```python
from build123d import *

# Parameters (mm, degrees)
F1_DEPTH = 63.5
F2_DEPTH = 25.4
F3_DEPTH = 7.9375
F5_R     = 6.35
F6_R     = 6.35
F7_R     = 6.35
F8_R     = 6.35


with BuildPart() as f1:
    # F0 (on Front) → F1 (new body, symmetric)
    with BuildSketch(Plane.XZ):
        Polygon((22.225, 9.525), (-41.275, 9.525), (-41.275, -9.525), (41.275, -9.525), (41.275, 9.525), align=None)
    extrude(amount=F1_DEPTH, both=True)

    # F0 (on Front) → F2 (join, symmetric)
    with BuildSketch(Plane.XZ):
        with BuildLine():
            Line((22.225, 27.32094), (22.225, 9.525))
            Line((22.225, 9.525), (41.275, 9.525))
            Line((41.275, 9.525), (41.275, 27.32094))
            ThreePointArc((41.275, 27.32094), (47.109768, 39.617662), (60.325, 42.8752))
            Line((60.325, 42.8752), (60.325, 61.857935))
            add(Edge.make_bspline(
                [(48.832623, 61.241094), (52.4914, 61.474881), (56.318798, 61.67946), (60.325, 61.857935)],
                knots=[108.446727, 108.446727, 108.446727, 108.446727, 114.871759, 114.871759, 114.871759, 114.871759], degree=3))
            ThreePointArc((48.832623, 61.241094), (29.670553, 48.876348), (22.225, 27.32094))
        make_face()
        with BuildLine():
            add(Edge.make_bspline(
                [(60.325, 61.857935), (60.837854, 61.880782), (61.353639, 61.903202), (61.872375, 61.9252)],
                knots=[114.871759, 114.871759, 114.871759, 114.871759, 115.69426, 115.69426, 115.69426, 115.69426], degree=3))
            Line((60.325, 61.857935), (60.325, 42.8752))
            Line((60.325, 42.8752), (85.725, 42.8752))
            Line((85.725, 42.8752), (85.725, 61.9252))
            Line((85.725, 61.9252), (61.872375, 61.9252))
        make_face()
    extrude(amount=F2_DEPTH, both=True)

    # F0 (on Front) → F3 (join, symmetric)
    with BuildSketch(Plane.XZ):
        with BuildLine():
            add(Edge.make_bspline(
                [(-41.275, 9.525), (-26.639564, 45.028193), (-12.923076, 57.295065), (48.832623, 61.241094)],
                knots=[0, 0, 0, 0, 108.446727, 108.446727, 108.446727, 108.446727], degree=3))
            Line((-41.275, 9.525), (22.225, 9.525))
            Line((22.225, 9.525), (22.225, 27.32094))
            ThreePointArc((22.225, 27.32094), (29.670553, 48.876348), (48.832623, 61.241094))
        make_face()
    extrude(amount=F3_DEPTH, both=True)

    # F0 (on Front) → F4 (revolve)
    with BuildSketch(Plane.XZ):
        Polygon((111.125, 66.675), (85.725, 66.675), (85.725, 61.9252), (85.725, 42.8752), (85.725, 38.1), (111.125, 38.1), align=None)
    revolve(axis=Axis((85.725, 0, 52.3875), (0, 0, 1)))

    # F5
    f5_edges = [f1.edges().sort_by_distance(p)[0] for p in [
        (41.275, -63.5, 0),
    ]]
    fillet(f5_edges, radius=F5_R)

    # F6
    f6_edges = [f1.edges().sort_by_distance(p)[0] for p in [
        (-41.275, -63.5, 0),
    ]]
    fillet(f6_edges, radius=F6_R)

    # F7
    f7_edges = [f1.edges().sort_by_distance(p)[0] for p in [
        (-41.275, 63.5, 0),
    ]]
    fillet(f7_edges, radius=F7_R)

    # F8
    f8_edges = [f1.edges().sort_by_distance(p)[0] for p in [
        (41.275, 63.5, 0),
    ]]
    fillet(f8_edges, radius=F8_R)


solid = f1.part
```
The listing builds one solid part. Answer for the finished solid, in the listing's coordinates (mm). A direction names the side the tool comes from. Give positions to 0.01 mm unless a question says otherwise; leave off trailing zeros. Loops run counter-clockwise (first coordinate to the right, second up) from the corner with the lowest first, then second, coordinate; pieces in that order, holes last. Notation, with made-up numbers: M 3,77 L 53,77 A21 ccw 53,85 Z; hole C 36.5,64 d8. An arc over 180 degrees is marked long. One line per item, written item: value.
Q1. Find the intervals of material crossed by line 1 (Z direction, x = 72, y = -22); line 2 (Y direction, x = -11, z = 31.5); line 3 (Y direction, x = 61, z = 53), in increasing order. Write a range as from..to.
Working result:
line 1: z = 42.88..61.93
line 2: y = -7.94..7.94
line 3: y = -25.4..25.4
Q2. For faces 1 (the face through (46, 25.4, 42)), 2 (the face through (29.87, 16.55, 49.13)), 3 (the face through (29.87, -16.79, 49.13)), 4 (the face through (46, -25.4, 42)), 5 (the face through (41.275, -1, 5)), determine the directions among +Z, -Z, +X, -X, +Y, -Y from which every point of the face is accessible in a straight line to the end or side of a thin tool.
Working result:
face 1: +Z, +X, -X, +Y
face 2: +Z, -X, +Y
face 3: +Z, -X, -Y
face 4: +Z, +X, -X, -Y
face 5: -Z, +X, +Y, -Y
Q3. Flat-ended cylindrical pins translate along their axes: P1, Ø15, axis at x = 94.5, y = -1.5, coming from the -Z side; P2, Ø6, axis at x = 24.5, y = -44, coming from the +Z side (3 decimals); P3, Ø15.5, axis at x = 69, z = 40.5, coming from the +Y side; P4, Ø19, axis at y = -16, z = 18, coming from the -X side (3 decimals). Find the tip coordinate at first contact, or state that the pin passes through.
Working result:
P1: stops at z = 38.1
P2: stops at z = 9.525
P3: stops at y = 25.4
P4: stops at x = -41.275
Q4. A cutting plane is placed at B-B on x = 80.5. Determine the outline of the cut face in (y, z) (3 decimals), then the cut area to 3 significant figures.
Working result:
outline: M -25.4,42.875 L -24.857,42.875 L -24.857,38.1 L 24.857,38.1 L 24.857,42.875 L 25.4,42.875 L 25.4,61.925 L 24.857,61.925 L 24.857,66.675 L -24.857,66.675 L -24.857,61.925 L -25.4,61.925 Z
area: 1,440 mm^2
Q5. A cutting plane is placed at C-C on y = -46. Determine the outline of the cut face in (x, z) (3 decimals), then the cut area to 3 significant figures.
Working result:
outline: M -41.275,-9.525 L 41.275,-9.525 L 41.275,9.525 L -41.275,9.525 Z
area: 1,570 mm^2
Q6. A cutting plane is placed at A-A on z = -3.5. Determine the outline of the cut face in (x, y) (3 decimals).
Working result:
outline: M -41.275,-57.15 A6.35 ccw -34.925,-63.5 L 34.925,-63.5 A6.35 ccw 41.275,-57.15 L 41.275,57.15 A6.35 ccw 34.925,63.5 L -34.925,63.5 A6.35 ccw -41.275,57.15 Z
